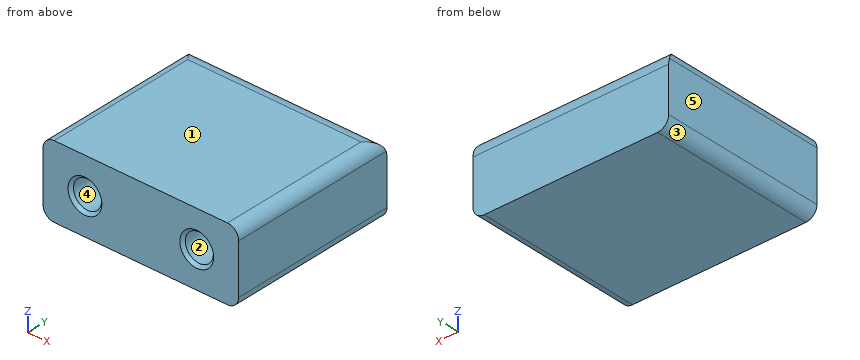
```python
from build123d import *

# Parameters (mm, degrees)
SKETCH1_W                   = 35
SKETCH1_H                   = 13
BOSS_EXTRUDE1_DEPTH         = 30
FILLET1_R                   = 2
FILLET2_R                   = 3
M6_TAPPED_HOLE1_D           = 5
M6_TAPPED_HOLE1_DEPTH       = 17
M6_TAPPED_HOLE1_CSINK_D     = 6.05
M6_TAPPED_HOLE1_CSINK_ANGLE = 90
M6_TAPPED_HOLE1_TIP         = 1.502151548


with BuildPart() as part:
    # Sketch1 → Boss-Extrude1 (new body)
    with BuildSketch(Plane(origin=(0, 0, 0), x_dir=(1, 0, 0), z_dir=(0, 1, 0))):
        Rectangle(SKETCH1_W, SKETCH1_H)
    extrude(amount=-BOSS_EXTRUDE1_DEPTH)

    # Fillet1
    fillet1_edges = [part.edges().sort_by_distance(p)[0] for p in [
        (17.5, -15, 6.5),
        (-17.5, -15, 6.5),
        (-17.5, -15, -6.5),
        (17.5, -15, -6.5),
    ]]
    fillet(fillet1_edges, radius=FILLET1_R)

    # Fillet2
    # the kernel refuses this fillet: 3 mm, written as the material it takes off along each edge
    with BuildSketch(Plane(origin=(-23, 0, 6.5), x_dir=(0, -1, 0), z_dir=(1, 0, 0))) as fillet2_piece_1:
        with BuildLine():
            CenterArc((FILLET2_R, FILLET2_R), FILLET2_R, 180, 90)
            Line((0, FILLET2_R), (0, 0))
            Line((0, 0), (FILLET2_R, 0))
        make_face()
    extrude(amount=46, mode=Mode.SUBTRACT)

    # M6 Tapped Hole1
    with Locations(Plane(origin=(0, -30, 0), x_dir=(-1, 0, 0), z_dir=(0, -1, 0))):
        with Locations((-10, 0), (10, 0)):
            CounterSinkHole(M6_TAPPED_HOLE1_D / 2, M6_TAPPED_HOLE1_CSINK_D / 2, depth=M6_TAPPED_HOLE1_DEPTH, counter_sink_angle=M6_TAPPED_HOLE1_CSINK_ANGLE)
            with Locations((0, 0, -(M6_TAPPED_HOLE1_DEPTH + M6_TAPPED_HOLE1_TIP / 2))):  # 118° drill point
                Cone(0, M6_TAPPED_HOLE1_D / 2, M6_TAPPED_HOLE1_TIP, mode=Mode.SUBTRACT)


solid = part.part
```
Design review of the part built by this model. Coordinates are the model's own, in mm. Face numbers are marked on the shaded views. A direction names the side the tool comes from. Give positions to 0.01 mm unless a question says otherwise; leave off trailing zeros. Write each loop counter-clockwise with the first axis right and the second up, starting at its lowest first coordinate (ties: lowest second). Pieces come first, ordered by that corner, then holes. Notation, with made-up numbers: (45.5, 71) - (97.5, 71) arc R16 ccw to (97.5, 91) - close; hole circle Ø6 at (-14.5, 4.25). An arc over 180 degrees is marked (long way). Return JSON: item names as keys, results as strings. Group by question number.
(1) To check wall thickness, follow probe 1 along Z at (x, y) = (-10, -23); probe 2 along X at (y, z) = (-22, 1); probe 3 along X at (y, z) = (-15.5, -0.5). State the ranges of each line that lie inside material, in increasing order.
(2) Machinability: for the marked faces 1 and 2, which of the approach directions +Z, -Z, +X, -X, +Y, -Y give a long, thin tool a straight path to every point of the face, cutting with its end or side? Answer none if there is none.
(3) Insertion check: pin 1 (6 mm diameter, centred on x = 10, z = 0, fed in from -Y) (3 decimals). The pin has a flat end and moves straight along its axis. Give the tip position at first contact, or say it passes through.
(4) Mouldability with a two-part tool opening along Z and no side actions: class the marked faces 3, 4 and 5 as +Z half, -Z half, draft (parallel to the pull), parting line (faces both ways), or undercut.
(5) We need section A-A, the plane y = -20.5. Give the boundary of the cut face in (x, z), then the cut area to 3 significant figures.
Reported:
{
 "1": {"probe 1": "z = -6.5 to -2.5, 2.5 to 6.5", "probe 2": "x = -17.5 to -12.29, -7.71 to 7.71, 12.29 to 17.5", "probe 3": "x = -17.5 to -12.45, -7.55 to 7.55, 12.45 to 17.5"},
 "2": {"face 1": "+Z, +X, -X, +Y, -Y", "face 2": "-Y"},
 "3": {"pin 1": "stops at y = -29.975"},
 "4": {"face 3": "-Z half", "face 4": "undercut", "face 5": "draft"},
 "5": {"outline": "(-17.5, -4.5) arc R2 ccw to (-15.5, -6.5) - (15.5, -6.5) arc R2 ccw to (17.5, -4.5) - (17.5, 4.5) arc R2 ccw to (15.5, 6.5) - (-15.5, 6.5) arc R2 ccw to (-17.5, 4.5) - close; hole circle Ø5 at (-10, 0); hole circle Ø5 at (10, 0)", "area": "412 mm2"}
}
